Design review of the part built by this model. Coordinates are the model's own, in mm. Coordinates: 2 decimals unless noted, no trailing zeros. Write each loop counter-clockwise with the first axis right and the second up, starting at its lowest first coordinate (ties: lowest second). Pieces come first, ordered by that corner, then holes. Notation, with made-up numbers: (4, -28) - (23, -28) arc R16 ccw to (23, 2) - close; hole circle Ø3 at (15.25, -2.75). An arc over 180 degrees is marked (long way). One line per item, written item: value.
from build123d import *

# Parameters (mm, degrees)
SKETCH1_W                     = 127
SKETCH1_H                     = 127
BOSS_EXTRUDE1_DEPTH           = 82.55
SKETCH2_R                     = 3.175
CUT_EXTRUDE1_DEPTH            = 83.55
LPATTERN1_COUNT               = 2
LPATTERN1_PITCH               = 31.75
LPATTERN1_COL_COUNT           = 2
LPATTERN1_COL_PITCH           = 31.75
LPATTERN2_COUNT               = 2
LPATTERN2_PITCH               = 31.75
LPATTERN2_COPY_1_SKETCH_R     = 3.175
LPATTERN2_COPY_1_DEPTH        = 83.55
LPATTERN2_COPY_2_SKETCH_R     = 3.175
LPATTERN2_COPY_2_DEPTH        = 83.55
LPATTERN2_COL_COUNT           = 2
LPATTERN2_COL_PITCH           = 31.75
LPATTERN2_COL_COPY_1_SKETCH_R = 3.175
LPATTERN2_COL_COPY_1_DEPTH    = 83.55
LPATTERN2_COL_COPY_2_SKETCH_R = 3.175
LPATTERN2_COL_COPY_2_DEPTH    = 83.55
SKETCH3_R                     = 3.175
CUT_EXTRUDE2_DEPTH            = 83.55


with BuildPart() as part:
    # Sketch1 → Boss-Extrude1 (new body)
    with BuildSketch(Plane.XY):
        Rectangle(SKETCH1_W, SKETCH1_H)
    extrude(amount=BOSS_EXTRUDE1_DEPTH)

    # Sketch2 → Cut-Extrude1 (cut, through all)
    with BuildSketch(Plane.XY.offset(82.55)):
        Circle(SKETCH2_R)
    cut_extrude1 = extrude(amount=-CUT_EXTRUDE1_DEPTH, mode=Mode.SUBTRACT)

    # LPattern1: Cut-Extrude1 ×2
    with Locations(*[(-i * LPATTERN1_PITCH, 0, 0) for i in range(1, LPATTERN1_COUNT)]):
        add(cut_extrude1, mode=Mode.SUBTRACT)

    # LPattern1 col: Cut-Extrude1 ×2
    with Locations(*[(i * LPATTERN1_COL_PITCH, 0, 0) for i in range(1, LPATTERN1_COL_COUNT)]):
        add(cut_extrude1, mode=Mode.SUBTRACT)

    # LPattern2: Cut-Extrude1 ×2
    with Locations(*[(0, -i * LPATTERN2_PITCH, 0) for i in range(1, LPATTERN2_COUNT)]):
        add(cut_extrude1, mode=Mode.SUBTRACT)

    # LPattern2 copy 1 sketch → LPattern2 copy 1 (cut, through all)
    with BuildSketch(Plane(origin=(-31.75, -31.75, 82.55), x_dir=(1, 0, 0), z_dir=(0, 0, 1))):
        Circle(LPATTERN2_COPY_1_SKETCH_R)
    extrude(amount=-LPATTERN2_COPY_1_DEPTH, mode=Mode.SUBTRACT)

    # LPattern2 copy 2 sketch → LPattern2 copy 2 (cut, through all)
    with BuildSketch(Plane(origin=(31.75, -31.75, 82.55), x_dir=(1, 0, 0), z_dir=(0, 0, 1))):
        Circle(LPATTERN2_COPY_2_SKETCH_R)
    extrude(amount=-LPATTERN2_COPY_2_DEPTH, mode=Mode.SUBTRACT)

    # LPattern2 col: Cut-Extrude1 ×2
    with Locations(*[(0, i * LPATTERN2_COL_PITCH, 0) for i in range(1, LPATTERN2_COL_COUNT)]):
        add(cut_extrude1, mode=Mode.SUBTRACT)

    # LPattern2 col copy 1 sketch → LPattern2 col copy 1 (cut, through all)
    with BuildSketch(Plane(origin=(-31.75, 31.75, 82.55), x_dir=(1, 0, 0), z_dir=(0, 0, 1))):
        Circle(LPATTERN2_COL_COPY_1_SKETCH_R)
    extrude(amount=-LPATTERN2_COL_COPY_1_DEPTH, mode=Mode.SUBTRACT)

    # LPattern2 col copy 2 sketch → LPattern2 col copy 2 (cut, through all)
    with BuildSketch(Plane(origin=(31.75, 31.75, 82.55), x_dir=(1, 0, 0), z_dir=(0, 0, 1))):
        Circle(LPATTERN2_COL_COPY_2_SKETCH_R)
    extrude(amount=-LPATTERN2_COL_COPY_2_DEPTH, mode=Mode.SUBTRACT)

    # Sketch3 → Cut-Extrude2 (cut, through all)
    with BuildSketch(Plane.XY.offset(82.55)):
        with Locations((-50.8, 50.8)):
            Circle(SKETCH3_R)
        with Locations((50.8, 50.8)):
            Circle(SKETCH3_R)
        with Locations((50.8, -50.8)):
            Circle(SKETCH3_R)
        with Locations((-50.8, -50.8)):
            Circle(SKETCH3_R)
    extrude(amount=-CUT_EXTRUDE2_DEPTH, mode=Mode.SUBTRACT)


solid = part.part
1. Wall thickness on line 1 along Y through (x, z) = (0, 19) (3 decimals); line 2 along Y through (x, z) = (-30, 77); line 3 along X through (y, z) = (50, 21): over which ranges is each line inside the solid? List them lowest first.
Answer block:
line 1: y = -63.5 to -34.925, -28.575 to -3.175, 3.175 to 28.575, 34.925 to 63.5
line 2: y = -63.5 to -34.4, -29.1 to -2.65, 2.65 to 29.1, 34.4 to 63.5
line 3: x = -63.5 to -53.87, -47.73 to 47.73, 53.87 to 63.5
2. Consider section C-C, the plane z = 75. Give the number of separate pieces and of enclosed holes in the cut face, then the cut area to 3 significant figures.
Answer block:
separate pieces: 1
enclosed holes: 13
area: 15,700 mm^2
3. Consider section B-B, the plane x = 0. Write out the cut boundary in (y, z) (3 decimals), then the cut area to 3 significant figures.
Answer block:
outline: (-63.5, 0) - (-34.925, 0) - (-34.925, 82.55) - (-63.5, 82.55) - close; (-28.575, 0) - (-3.175, 0) - (-3.175, 82.55) - (-28.575, 82.55) - close; (3.175, 0) - (28.575, 0) - (28.575, 82.55) - (3.175, 82.55) - close; (34.925, 0) - (63.5, 0) - (63.5, 82.55) - (34.925, 82.55) - close
area: 8,910 mm^2
4. Mouldability with a two-part tool opening along Y and no side actions: class faces 1 (the face through (13, 1, 0)), 2 (the face through (-1, 63.5, 41)), 3 (the face through (-1, -63.5, 41)), 4 (the face through (-34.92, 0.14, 41.85)) as released by +Y, released by -Y, zero draft, split by the parting line, or undercut.
Answer block:
face 1: zero draft
face 2: released by +Y
face 3: released by -Y
face 4: undercut
5. Consider section A-A, the plane x = 50.8. Write out the cut boundary in (y, z) (3 decimals).
Answer block:
outline: (-63.5, 0) - (-53.975, 0) - (-53.975, 82.55) - (-63.5, 82.55) - close; (-47.625, 0) - (47.625, 0) - (47.625, 82.55) - (-47.625, 82.55) - close; (53.975, 0) - (63.5, 0) - (63.5, 82.55) - (53.975, 82.55) - close
6. Insertion check: pin 1 Ø6 at (x, y) = (23.5, -36.5) entering from -Z. The pin has a flat end and moves straight along its axis. Give the tip position at first contact, or say it passes through.
Answer block:
pin 1: stops at z = 0
